Could you check a few things on this model? Use its own coordinates, in mm. A direction names the side the tool comes from. Coordinates: 2 decimals unless noted, no trailing zeros. Write each loop counter-clockwise with the first axis right and the second up, starting at its lowest first coordinate (ties: lowest second). Pieces come first, ordered by that corner, then holes.
```python
from build123d import *

# Parameters (mm, degrees)
SKETCH_1_R               = 30
EXTRUDE_1_DEPTH          = 25
EXTRUDE_2_DEPTH          = 10
EXTRUDE_3_DEPTH          = 10
CUT_EXTRUDE_1_DEPTH      = 10
SKETCH_5_R               = 1.375
CUT_EXTRUDE_2_DEPTH      = 3
SKETCH_7_R               = 28
CUT_EXTRUDE_4_DEPTH      = 17
SKETCH_8_R               = 1.225
CUT_EXTRUDE_5_DEPTH      = 22
SKETCH_10_R              = 3
CUT_EXTRUDE_6_DEPTH      = 50.244289121
CUT_EXTRUDE_START        = -17
CUT_EXTRUDE_8_DEPTH      = 17
CUT_EXTRUDE_START_2      = -5
SKETCH_14_R              = 30
CUT_EXTRUDE_9_DEPTH      = 5
SKETCH_11_R              = 2.25
CUT_EXTRUDE_10_DEPTH     = 2.5
PATTERN_CIRCULAR_1_COUNT = 4
CUT_EXTRUDE_11_DEPTH     = 5


with BuildPart() as part:
    # Sketch 1 → Extrude 1 (new body)
    with BuildSketch(Plane.XY):
        Circle(SKETCH_1_R)
    extrude(amount=EXTRUDE_1_DEPTH)

    # Sketch 2 → Extrude 2 (add)
    with BuildSketch(Plane(origin=(0, 0, 0), x_dir=(-1, 0, 0), z_dir=(0, 0, -1))):
        with BuildLine():
            Line((12.5, 30), (0, 30))
            ThreePointArc((0, 30), (6.397131834, 29.310010309), (12.5, 27.271780287))
            Line((12.5, 27.271780287), (12.5, 30))
        make_face()
        with BuildLine():
            Line((0, 30), (-12.5, 30))
            Line((-12.5, 30), (-12.5, 27.271780287))
            ThreePointArc((-12.5, 27.271780287), (-6.397131834, 29.310010309), (0, 30))
        make_face()
    extrude(amount=-EXTRUDE_2_DEPTH)

    # Sketch 3 → Extrude 3 (add)
    with BuildSketch(Plane.XY.offset(10)):
        with BuildLine():
            Line((-12.5, 30), (-12.5, 27.271780287))
            ThreePointArc((-12.5, 27.271780287), (-6.397131834, 29.310010309), (0, 30))
            Line((0, 30), (-12.5, 30))
        make_face()
        with BuildLine():
            ThreePointArc((0, 30), (6.397131834, 29.310010309), (12.5, 27.271780287))
            Line((12.5, 27.271780287), (12.5, 30))
            Line((12.5, 30), (0, 30))
        make_face()
    extrude(amount=EXTRUDE_3_DEPTH)

    # Sketch 4 → Cut-Extrude 1 (cut)
    with BuildSketch(Plane(origin=(0, 0, 0), x_dir=(-1, 0, 0), z_dir=(0, 0, -1))):
        with BuildLine():
            Line((-12.5, 30), (-12.5, 27.271780287))
            ThreePointArc((-12.5, 27.271780287), (-6.397131834, 29.310010309), (0, 30))
            Line((0, 30), (-12.5, 30))
        make_face()
        with BuildLine():
            ThreePointArc((0, 30), (6.397131834, 29.310010309), (12.5, 27.271780287))
            Line((12.5, 27.271780287), (12.5, 30))
            Line((12.5, 30), (0, 30))
        make_face()
    extrude(amount=-CUT_EXTRUDE_1_DEPTH, mode=Mode.SUBTRACT)

    # Sketch 5 → Cut-Extrude 2 (cut)
    with BuildSketch(Plane(origin=(0, 30, 0), x_dir=(1, 0, 0), z_dir=(0, 1, 0))):
        with Locations(Location((-3.75, -16.5, 0), (0, 0, 270))):
            Circle(SKETCH_5_R)
        with Locations(Location((3.75, -16.5, 0), (0, 0, 270))):
            Circle(SKETCH_5_R)
    extrude(amount=-CUT_EXTRUDE_2_DEPTH, mode=Mode.SUBTRACT)

    # Sketch 7 → Cut-Extrude 4 (cut)
    with BuildSketch(Plane.XY.offset(25)):
        Circle(SKETCH_7_R)
    extrude(amount=-CUT_EXTRUDE_4_DEPTH, mode=Mode.SUBTRACT)

    # Sketch 8 → Cut-Extrude 5 (cut)
    with BuildSketch(Plane(origin=(0, 0, 0), x_dir=(-1, 0, 0), z_dir=(0, 0, -1))):
        with Locations((0, -19.25)):
            Circle(SKETCH_8_R)
        with Locations((-19.25, 0)):
            Circle(SKETCH_8_R)
        with Locations((0, 19.25)):
            Circle(SKETCH_8_R)
        with Locations((19.25, 0)):
            Circle(SKETCH_8_R)
    extrude(amount=-CUT_EXTRUDE_5_DEPTH, mode=Mode.SUBTRACT)

    # Sketch 10 → Cut-Extrude 6 (cut, through all)
    with BuildSketch(Plane(origin=(0, 0, 0), x_dir=(-1, 0, 0), z_dir=(0, 0, -1))):
        Circle(SKETCH_10_R)
    extrude(amount=-CUT_EXTRUDE_6_DEPTH, mode=Mode.SUBTRACT)

    # Sketch 13 → Cut-Extrude 8 (cut)
    with BuildSketch(Plane.XY.offset(25).offset(CUT_EXTRUDE_START)):
        with BuildLine():
            Line((14.928300859, 4.321699141), (25.842896765, 15.236295048))
            ThreePointArc((25.842896765, 15.236295048), (21.213203436, 21.213203436), (15.236295048, 25.842896765))
            Line((15.236295048, 25.842896765), (4.321699141, 14.928300859))
            Line((4.321699141, 14.928300859), (14.928300859, 4.321699141))
        make_face()
    extrude(amount=CUT_EXTRUDE_8_DEPTH, mode=Mode.SUBTRACT)

    # Sketch 14 → Cut-Extrude 9 (cut)
    with BuildSketch(Plane.XY.offset(25).offset(CUT_EXTRUDE_START_2)):
        with Locations(Location((0, 0, 0), (0, 0, 114.624318352))):
            Circle(SKETCH_14_R)
    extrude(amount=CUT_EXTRUDE_9_DEPTH, mode=Mode.SUBTRACT)

    # Sketch 11 → Cut-Extrude 10 (cut)
    with BuildSketch(Plane(origin=(0, 0, 0), x_dir=(-1, 0, 0), z_dir=(0, 0, -1))):
        with Locations((0, 19.25)):
            Circle(SKETCH_11_R)
    cut_extrude_10 = extrude(amount=-CUT_EXTRUDE_10_DEPTH, mode=Mode.SUBTRACT)

    # Pattern Circular 1: Cut-Extrude 10 ×4 about axis
    pattern_circular_1_axis = Axis((0, 0, 0), (0, 0, 1))
    for i in range(1, PATTERN_CIRCULAR_1_COUNT):
        add(cut_extrude_10.rotate(pattern_circular_1_axis, i * 360 / PATTERN_CIRCULAR_1_COUNT), mode=Mode.SUBTRACT)

    # Sketch 17 → Cut-Extrude 11 (cut)
    with BuildSketch(Plane(origin=(0, 0, 0), x_dir=(-1, 0, 0), z_dir=(0, 0, -1))):
        Polygon((5.77, 0), (2.885, 4.99696658), (-2.885, 4.99696658), (-5.77, 0), (-2.885, -4.99696658), (2.885, -4.99696658), align=None)
    extrude(amount=-CUT_EXTRUDE_11_DEPTH, mode=Mode.SUBTRACT)


solid = part.part
```
1. I want a section at B-B on x = 3.75. Please give me the cut outline in (y, z) (3 decimals), plus the area to 3 significant figures.
Verdict:
outline: (-29.765, 0) - (-3.499, 0) - (-3.499, 5) - (3.499, 5) - (3.499, 0) - (29.765, 0) - (29.765, 10) - (30, 10) - (30, 15.125) - (27.748, 15.125) - (27.748, 8) - (-27.748, 8) - (-27.748, 20) - (-29.765, 20) - close; (27.748, 17.875) - (30, 17.875) - (30, 20) - (27.748, 20) - close
area: 486 mm2
2. On a 3-axis mill with a long thin cutter (end or side, diameter ignored), from which of +Z, -Z, +X, -X, +Y, -Y can I reach the whole of each face in a straight line? I mean faces 4 (the face through (-2.5, 2.3, 5)), 5 (the face through (5.113, 28.781, 16.321)), 6 (the face through (-20.578, -18.988, 14.084)), 7 (the face through (-9, 29, 10)). Say none if no direction works.
Verdict:
face 4: -Z
face 5: +Y
face 6: +Z
face 7: -Z, -X, +Y
3. I want a section at D-D on y = 6.5. Please give me the cut outline in (x, z), plus the area to 3 significant figures.
Verdict:
outline: (-29.29, 0) - (29.29, 0) - (29.29, 20) - (27.24, 20) - (27.24, 8) - (-27.24, 8) - (-27.24, 20) - (-29.29, 20) - close
area: 518 mm2
4. For pin 1 (1.6 mm diameter, centred on x = -3.75, z = 16.5, fed in from -Y); pin 2 (3 mm diameter, centred on x = -18, y = -10.5, fed in from +Z); pin 3 (2 mm diameter, centred on x = -18.5, y = 0.5, fed in from -Z); pin 4 (2 mm diameter, centred on x = -19.25, y = 0, fed in from -Z), each with a flat end and sliding along its axis, tell me the tip position at first contact or that it passes through.
Verdict:
pin 1: stops at y = -29.85
pin 2: stops at z = 8
pin 3: stops at z = 2.5
pin 4: passes through
5. If we mould it in two halves opening along X, with no side actions, what happens to faces 1 (the face through (12.5, 29, 15)), 2 (the face through (0.159, 20.465, 5.212)), 3 (the face through (-6, 0, 0))? For each: pulls with the +X half, pulls with the -X half, needs draft (parallel to the pull), parting line crosses it, or undercut.
Verdict:
face 1: pulls with the +X half
face 2: undercut
face 3: needs draft
6. I want a section at A-A on z = 7. Please give me the cut outline in (x, y) (3 decimals), plus the area to 3 significant figures.
Verdict:
outline: circle Ø60 at (0, 0); hole circle Ø2.45 at (-19.25, 0); hole circle Ø6 at (0, 0); hole circle Ø2.45 at (0, -19.25); hole circle Ø2.45 at (0, 19.25); hole circle Ø2.45 at (19.25, 0)
area: 2,780 mm2
7. Please list where these lines run through material, in increasing order: line 1 along X through (y, z) = (28.4, 16.5) (3 decimals); line 2 along Y through (x, z) = (0.5, 14); line 3 along Y through (x, z) = (-7.5, 8.25).
Verdict:
line 1: x = -12.5 to -5.125, -2.375 to 2.375, 5.125 to 12.5
line 2: y = -30 to -28, 28 to 30
line 3: y = -29.05 to -26.98, 26.98 to 29.05
